Design review of the part shown in the three views and the two pictorial views. Dimensions are in mm from the part's minimum x, y and z. A direction names the side the tool comes from. Give positions to 0.01 mm unless a question says otherwise; leave off trailing zeros. Loops run counter-clockwise (first coordinate to the right, second up) from the corner with the lowest first, then second, coordinate; pieces in that order, holes last. Notation, with made-up numbers: (-28, 80.5) - (13, 80.5) arc R18 cw to (13, 97.5) - close; hole circle Ø3 at (77.5, 8). An arc over 180 degrees is marked (long way). Return JSON: item names as keys, results as strings. Group by question number.
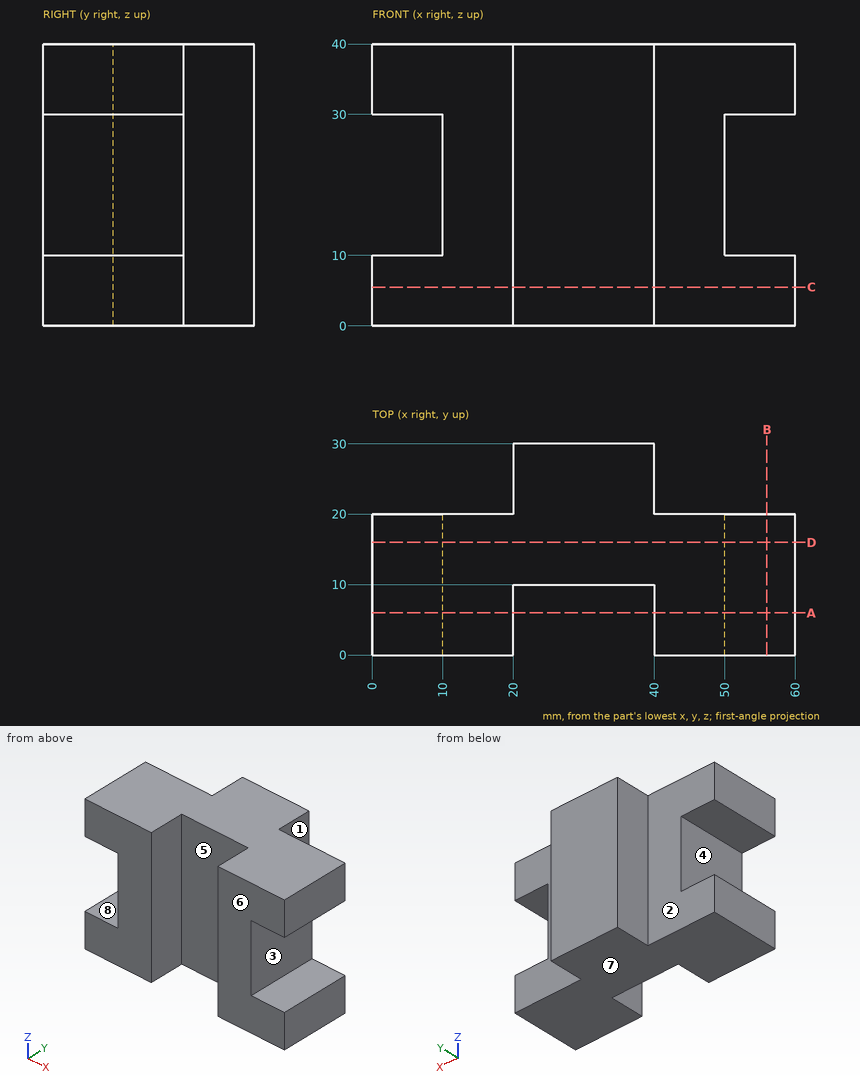
Item 1: For P1, Ø5, axis at y = 26, z = 25.5, coming from the +X side; P2, Ø22, axis at x = 6, z = 16.5, coming from the +Y side; P3, Ø3, axis at y = 5, z = 17, coming from the -X side, all flat-tipped, find the tip position at first contact; note any pin that passes through.
Item 2: Take a section at A-A (y = 6). State the section outline as (x, z) points.
Item 3: Take a section at B-B (x = 56). State the section outline as (y, z) points, then the cut area to 3 significant figures.
Item 4: Take a section at D-D (y = 16). State the section outline as (x, z) points.
Item 5: Tool access review of the marked faces 1, 2, 3, 4 and 5: name each direction out of +Z, -Z, +X, -X, +Y, -Y from which nothing blocks a thin tool from reaching the whole face with its end or side.
Item 6: Take a section at C-C (z = 5.5). State the section outline as (x, y) points.
Item 7: For L1, parallel to X at y = 2.5, z = 31.5; L2, parallel to X at y = 7.25, z = 18.5; L3, parallel to Z at x = 55, y = 13, list the stretches that pass through material, from the lowest coordinate up. Write a range as from..to.
Item 8: Mouldability with a two-part tool opening along Z and no side actions: class the marked faces 6, 7 and 8 as +Z half, -Z half, draft (parallel to the pull), parting line (faces both ways), or undercut.
Check sheet entries:
{
 "1": {"P1": "stops at x = 40", "P2": "stops at y = 20", "P3": "stops at x = 10"},
 "2": {"outline": "(0, 0) - (20, 0) - (20, 40) - (0, 40) - (0, 30) - (10, 30) - (10, 10) - (0, 10) - close; (40, 0) - (60, 0) - (60, 10) - (50, 10) - (50, 30) - (60, 30) - (60, 40) - (40, 40) - close"},
 "3": {"outline": "(0, 0) - (20, 0) - (20, 10) - (0, 10) - close; (0, 30) - (20, 30) - (20, 40) - (0, 40) - close", "area": "400 mm^2"},
 "4": {"outline": "(0, 0) - (60, 0) - (60, 10) - (50, 10) - (50, 30) - (60, 30) - (60, 40) - (0, 40) - (0, 30) - (10, 30) - (10, 10) - (0, 10) - close"},
 "5": {"face 1": "+Z, -Z, +X, +Y", "face 2": "+Z, -Z, -X, +Y", "face 3": "+X, +Y, -Y", "face 4": "-X, +Y, -Y", "face 5": "+Z, -Z, -Y"},
 "6": {"outline": "(0, 0) - (20, 0) - (20, 10) - (40, 10) - (40, 0) - (60, 0) - (60, 20) - (40, 20) - (40, 30) - (20, 30) - (20, 20) - (0, 20) - close"},
 "7": {"L1": "x = 0..20, 40..60", "L2": "x = 10..20, 40..50", "L3": "z = 0..10, 30..40"},
 "8": {"face 6": "draft", "face 7": "-Z half", "face 8": "undercut"}
}
